from build123d import *

# Parameters (mm, degrees)
F1_DEPTH  = 15
F3_DEPTH  = 20
F5_DEPTH  = 20
F14_DEPTH = 20
F15_DEPTH = 20
F16_DEPTH = 20
F17_DEPTH = 20
F18_DEPTH = 20
F19_DEPTH = 20
F20_DEPTH = 20
F21_DEPTH = 20
F23_R     = 30
F23_R_2   = 27
F24_DEPTH = 13
F26_R     = 1
F27_DEPTH = 8


# Not quite as in the source:
# - a fillet or chamfer that OpenCascade refuses, or shapes differently, is made with other operations: its cross-section is extruded or revolved along the edge and cut away or added


with BuildPart() as f1:
    # F0 (on Top) → F1 (new body)
    with BuildSketch(Plane.XY):
        Polygon((7.5, -2.4368977217), (7.5, 2.4368977217), (4.6352549156, 6.3798810626), (0, 7.8859666818), (-4.6352549156, 6.3798810626), (-7.5, 2.4368977217), (-7.5, -2.4368977217), (-4.6352549156, -6.3798810626), (0, -7.8859666818), (4.6352549156, -6.3798810626), align=None)
    extrude(amount=F1_DEPTH)

    # F2 (on face) → F3 (join)
    with BuildSketch(Plane(origin=(-2.3176274578, -7.1329238722, 0), x_dir=(0.9510565163, -0.3090169944, 0), z_dir=(-0.3090169944, -0.9510565163, 0))):
        Polygon((2.4368977217, 12.0518097386), (-2.4368977217, 0), (2.4368977217, 0), align=None)
    extrude(amount=F3_DEPTH)

    # F4 (on face) → F5 (join)
    with BuildSketch(Plane(origin=(-6.0676274578, -4.4083893922, 0), x_dir=(0.5877852523, -0.8090169944, 0), z_dir=(-0.8090169944, -0.5877852523, 0))):
        Polygon((2.4368977217, 12.0518097386), (-2.4368977217, 0), (2.4368977217, 0), align=None)
    extrude(amount=F5_DEPTH)

    # F13 (on face) → F14 (join)
    with BuildSketch(Plane(origin=(2.3176274578, -7.1329238722, 0), x_dir=(0.9510565163, 0.3090169944, 0), z_dir=(0.3090169944, -0.9510565163, 0))):
        Polygon((2.4368977217, 12.0518097386), (-2.4368977217, 0), (2.4368977217, 0), align=None)
    extrude(amount=F14_DEPTH)

    # F12 (on face) → F15 (join)
    with BuildSketch(Plane(origin=(6.0676274578, -4.4083893922, 0), x_dir=(0.5877852523, 0.8090169944, 0), z_dir=(0.8090169944, -0.5877852523, 0))):
        Polygon((2.4368977217, 12.0518097386), (-2.4368977217, 0), (2.4368977217, 0), align=None)
    extrude(amount=F15_DEPTH)

    # F11 (on face) → F16 (join)
    with BuildSketch(Plane.YZ.offset(7.5)):
        Polygon((2.4368977217, 12.0518097386), (-2.4368977217, 0), (2.4368977217, 0), align=None)
    extrude(amount=F16_DEPTH)

    # F10 (on face) → F17 (join)
    with BuildSketch(Plane(origin=(6.0676274578, 4.4083893922, 0), x_dir=(-0.5877852523, 0.8090169944, 0), z_dir=(0.8090169944, 0.5877852523, 0))):
        Polygon((2.4368977217, 12.0518097386), (-2.4368977217, 0), (2.4368977217, 0), align=None)
    extrude(amount=F17_DEPTH)

    # F9 (on face) → F18 (join)
    with BuildSketch(Plane(origin=(2.3176274578, 7.1329238722, 0), x_dir=(-0.9510565163, 0.3090169944, 0), z_dir=(0.3090169944, 0.9510565163, 0))):
        Polygon((2.4368977217, 12.0518097386), (-2.4368977217, 0), (2.4368977217, 0), align=None)
    extrude(amount=F18_DEPTH)

    # F8 (on face) → F19 (join)
    with BuildSketch(Plane(origin=(-2.3176274578, 7.1329238722, 0), x_dir=(-0.9510565163, -0.3090169944, 0), z_dir=(-0.3090169944, 0.9510565163, 0))):
        Polygon((2.4368977217, 12.0518097386), (-2.4368977217, 0), (2.4368977217, 0), align=None)
    extrude(amount=F19_DEPTH)

    # F7 (on face) → F20 (join)
    with BuildSketch(Plane(origin=(-6.0676274578, 4.4083893922, 0), x_dir=(-0.5877852523, -0.8090169944, 0), z_dir=(-0.8090169944, 0.5877852523, 0))):
        Polygon((2.4368977217, 12.0518097386), (-2.4368977217, 0), (2.4368977217, 0), align=None)
    extrude(amount=F20_DEPTH)

    # F6 (on face) → F21 (join)
    with BuildSketch(Plane(origin=(-7.5, 0, 0), x_dir=(0, -1, 0), z_dir=(-1, 0, 0))):
        Polygon((2.4368977217, 12.0518097386), (-2.4368977217, 0), (2.4368977217, 0), align=None)
    extrude(amount=F21_DEPTH)

    # F23 (on face) → F24 (join)
    with BuildSketch(Plane.XY):
        Circle(F23_R)
        Circle(F23_R_2, mode=Mode.SUBTRACT)
    extrude(amount=F24_DEPTH)

    # F25: fillet of radius 3.5 on 1 edges, made by hand

    # F25_s1 → F25_t2 (revolve, cut)
    with BuildSketch(Plane.XZ):
        with BuildLine():
            ThreePointArc((27, 13), (29.1457513111, 11.8271862323), (30, 9.5358983849))
            Line((30, 9.5358983849), (30, 13))
            Line((30, 13), (27, 13))
        make_face()
    revolve(axis=Axis((0, 0, 13), (0, 0, 1)), mode=Mode.SUBTRACT)

    # F26 (on face) → F27 (join)
    with BuildSketch(Plane.XY):
        Circle(F26_R)
    extrude(amount=F27_DEPTH)


solid = f1.part
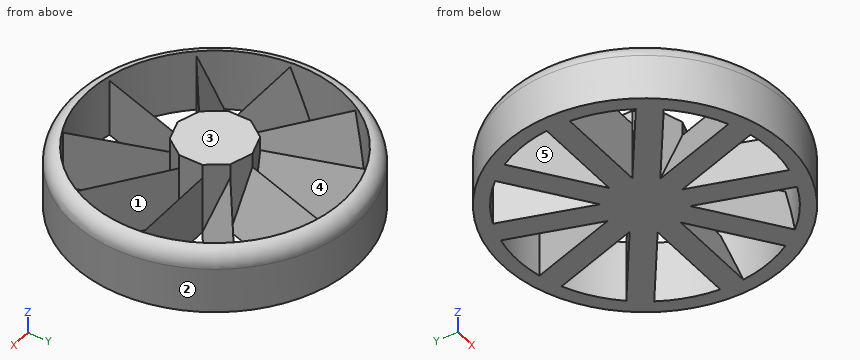
Read the model definition and answer for the solid it produces. Units are mm, in the model's axes. Face numbers are marked on the shaded views. A direction names the side the tool comes from. Give positions to 0.01 mm unless a question says otherwise; leave off trailing zeros. Write each loop counter-clockwise with the first axis right and the second up, starting at its lowest first coordinate (ties: lowest second). Pieces come first, ordered by that corner, then holes. Notation, with made-up numbers: (-11, -39.75) - (37, -39.75) arc R10 cw to (37, -33.75) - close; hole circle Ø8 at (42.25, 43). An arc over 180 degrees is marked (long way). Answer in a Markdown table with one row per item. Add a question column.
Item 1: Section A-A, the plane y = 0 is taken. Write down the section's boundary in (x, z).
Item 2: Section B-B, the plane y = -23.5 is taken. Count the separate pieces of the cut face and the enclosed holes in it, and give its area (3 significant figures).
Item 3: A tool of negligible diameter and unlimited length cuts with its end or side. For the marked faces 4 and 5, from which of +Z, -Z, +X, -X, +Y, -Y can it reach the whole face along a straight path? Write none if from no direction.
Item 4: Determine the mould class of the marked faces 1, 2 and 3 for opening direction Y: pulls with the +Y half, pulls with the -Y half, needs draft (parallel to the pull), parting line crosses it, or undercut.
Item 5: Flat-ended cylindrical pins translate along their axes: P1, Ø12, axis at x = -15, y = 20.5, coming from the +Z side; P2, Ø1.5, axis at x = 13, z = 7.5, coming from the -Y side (3 decimals); P3, Ø1, axis at y = -9, z = 4, coming from the -X side; P4, Ø4, axis at y = -0.5, z = 7, coming from the -X side. Find the tip coordinate at first contact, or state that the pin passes through.
Item 6: Find the intervals of material crossed by L1, parallel to Y at x = 23, z = 10.5; L2, parallel to X at y = -4, z = 2.5; L3, parallel to Y at x = 23.5, z = 4.75, in increasing order.
Recorded:
| question | item | result |
|---|---|---|
| 1 | outline | (-30, 0) - (30, 0) - (30, 9.54) arc R3.5 ccw to (27, 13) - (27, 6.03) - (7.5, 6.03) - (7.5, 15) - (-7.5, 15) - (-7.5, 6.03) - (-27, 6.03) - (-27, 13) arc R3.5 ccw to (-30, 9.54) - close |
| 2 | separate pieces | 4 |
| 2 | enclosed holes | 0 |
| 2 | area | 192 mm2 |
| 3 | face 4 | +Z |
| 3 | face 5 | +Z, -Z |
| 4 | face 1 | undercut |
| 4 | face 2 | parting line crosses it |
| 4 | face 3 | needs draft |
| 5 | P1 | stops at z = 13 |
| 5 | P2 | stops at y = -27.385 |
| 5 | P3 | stops at x = -28.77 |
| 5 | P4 | stops at x = -30 |
| 6 | L1 | y = -19.05 to -13.7, 1.81 to 2.44, 14.14 to 19.05 |
| 6 | L2 | x = -29.73 to -26.7, -7.93 to 9.65, 26.7 to 29.73 |
| 6 | L3 | y = -18.65 to -13.29, -0.52 to 2.44, 13.29 to 18.65 |
